Build history of the part. All positions in model axes, mm. A direction names the side the tool comes from. Give positions to 0.01 mm unless a question says otherwise; leave off trailing zeros. Write each loop counter-clockwise with the first axis right and the second up, starting at its lowest first coordinate (ties: lowest second). Pieces come first, ordered by that corner, then holes. Notation, with made-up numbers: (-18, 66) -> (-11, 66) arc R21 cw to (-11, 81) -> close; hole circle Ø7 at (56.5, 64.25). An arc over 180 degrees is marked (long way). Put each result on its own line as item: value. Start each with the question number.
Item 1: Slice it at D-D, the plane x = -12. List the corners of the cut face in (y, z).
Item 2: Tool access for faces 1 (the flat face through (-10.6, 48.1, 2)), 2 (the cylindrical face through (10.28, 45.89, -4.93)), 3 (the cylindrical face through (-29.68, 56.1, -0.87)): list every direction of +Z, -Z, +X, -X, +Y, -Y with a clear straight run to the whole face (end or side of a thin tool).
Item 3: Flat gauge pins, fed straight in: pin 1 Ø7.5 at (x, y) = (-45, 53.5) entering from -Z; pin 2 Ø12 at (y, z) = (23, -4.5) entering from -X; pin 3 Ø4 at (y, z) = (47.5, 6.5) entering from +X; pin 4 Ø2 at (x, y) = (-35.84, 7.78) entering from -Z. Where does each tip first touch, or does it go through?
Item 4: Slice it at B-B, the plane z = -6.5. Give the number of separate pieces and of enclosed holes in the cut face, plus the area to 3 significant figures.
Item 5: Slice it at C-C, the plane y = 42.25. List the corners of the cut face in (x, z).
Item 6: Slice it at A-A, the plane x = -25. List the corners of the cut face in (y, z).
Item 7: Two-plate mould, pull along X, no slides. Class faces 4 (the cylindrical face through (24.295, 39.077, 1.479)), 5 (the flat face through (0, 58, -7)), 6 (the flat face through (48.31, 28.36, 5.07)): pulls with the +X half, pulls with the -X half, needs draft (parallel to the pull), parting line crosses it, or undercut.
Item 8: Drill centre lines: line 1 along X through (y, z) = (8, -7.75); line 2 along Z through (x, y) = (2.5, 16.5); line 3 along Z through (x, y) = (23.5, 20). Where is each one in solid material? Low to high.
```python
from build123d import *

# Parameters (mm, degrees)
BOSS_EXTRUDE2_DEPTH              = 10
FILLET1_R                        = 7.777777778
SKETCH11_R                       = 2.425
SKETCH11_R_2                     = 4
BOSS_EXTRUDE3_DEPTH              = 10
CHAMFER1_SIZE                    = 0.699268119
CHAMFER1_SIZE_2                  = 10
SKETCH11_4_R                     = 3.5
SKETCH11_4_R_2                   = 2.425
BOSS_EXTRUDE4_DEPTH              = 1.5
CBORE_FOR_M3_SHCS2_D             = 3.6
CBORE_FOR_M3_SHCS2_CBORE_D       = 6.5
CBORE_FOR_M3_SHCS2_CBORE_DEPTH   = 8
CUT_EXTRUDE4_DEPTH               = 81.942358333
SKETCH31_W                       = 55
SKETCH31_H                       = 2
BOSS_EXTRUDE5_DEPTH              = 15
FILLET2_R                        = 5
CBORE_FOR_M3_SHCS3_OUTLINE_R     = 1.8
CBORE_FOR_M3_SHCS3_DEPTH         = 10
CBORE_FOR_M3_SHCS3_2_OUTLINE_R   = 3.25
CBORE_FOR_M3_SHCS3_2_OUTLINE_R_2 = 1.8
CBORE_FOR_M3_SHCS3_2_DEPTH       = 3
M3_CLEARANCE_HOLE4_D             = 3.6
SKETCH43_R                       = 4
BOSS_EXTRUDE6_DEPTH              = 10
CBORE_START                      = 2
CBORE_FOR_M3_SHCS4_OUTLINE_R     = 3.25
CBORE_FOR_M3_SHCS4_DEPTH         = 8
CBORE_START_2                    = -10
CBORE_FOR_M3_SHCS4_2_OUTLINE_R   = 1.8
CBORE_FOR_M3_SHCS4_2_DEPTH       = 12


# Read off the part's stored shape, not the designer's step: CBORE for M3 SHCS3, CBORE for M3 SHCS4
with BuildPart() as part:
    # Sketch9 → Boss-Extrude2 (new body)
    with BuildSketch(Plane.XY):
        Polygon((0, 0), (0, 59.5), (-56, 59.5), (-42, 0), align=None)
    boss_extrude2 = extrude(amount=BOSS_EXTRUDE2_DEPTH)

    # Mirror2: Boss-Extrude2 across plane
    add(boss_extrude2.mirror(Plane(origin=(0, 0, 10), x_dir=(0, 0, 1), z_dir=(-1, 0, 0))))

    # Fillet1
    fillet1_edges = [part.edges().sort_by_distance(p)[0] for p in [
        (42, 0, 5),
        (56, 59.5, 5),
        (-42, 0, 5),
        (-56, 59.5, 5),
    ]]
    fillet(fillet1_edges, radius=FILLET1_R)

    # Sketch11 → Boss-Extrude3 (add)
    with BuildSketch(Plane(origin=(0, 0, 0), x_dir=(-1, 0, 0), z_dir=(0, 0, -1))):
        with Locations(Location((-43.410908409, 54.412250943, 0), (0, 0, 180))):
            Circle(SKETCH11_R)
        with Locations(Location((-35.839885988, 7.777777778, 0), (0, 0, 180))):
            Circle(SKETCH11_R_2)
    boss_extrude3 = extrude(amount=BOSS_EXTRUDE3_DEPTH)

    # Chamfer1
    # the kernel refuses this chamfer: 10, 0.699268119 mm, written as the material it takes off along each edge
    with BuildSketch(Plane(origin=(-35.839885988, 0, 10), x_dir=(0, 0.8766829747338895, 0.48106856248536783), z_dir=(1, 0, 0))) as chamfer1_piece_1:
        Polygon((CHAMFER1_SIZE * 0.876682975279, -CHAMFER1_SIZE * 0.481068562785), (-CHAMFER1_SIZE_2 * 0.481068562485, -CHAMFER1_SIZE_2 * 0.876682974734), (0, 0), align=None)
    extrude(amount=71.679771977, mode=Mode.SUBTRACT)
    with BuildSketch(Plane(origin=(35.839885988, 7.777777778, 10), x_dir=(0, -1, 0), z_dir=(-1, 0, 0))) as chamfer1_piece_2:
        Polygon((7.777777778 - CHAMFER1_SIZE, 0), (7.777777778, -CHAMFER1_SIZE_2), (7.777777778, 0), align=None)
    revolve(axis=Axis((35.839885988, 7.777777778, 10), (0, 0, 1)), revolution_arc=76.759480085, mode=Mode.SUBTRACT)
    with BuildSketch(Plane(origin=(-35.839885988, 7.777777778, 10), x_dir=(0, -1, 0), z_dir=(1, 0, 0))) as chamfer1_piece_3:
        Polygon((7.777777778 - CHAMFER1_SIZE, 0), (7.777777778, CHAMFER1_SIZE_2), (7.777777778, 0), align=None)
    revolve(axis=Axis((-35.839885988, 7.777777778, 10), (0, 0, -1)), revolution_arc=76.759480085, mode=Mode.SUBTRACT)
    with BuildSketch(Plane(origin=(53.75077769, 49.940805182, 10), x_dir=(-0.8533782587917171, 0.2007948844215805, 0.4810685624853707), z_dir=(-0.2290393337255473, -0.973417168333576, 0))) as chamfer1_piece_4:
        Polygon((CHAMFER1_SIZE * 0.876682975279, CHAMFER1_SIZE * 0.481068562785), (-CHAMFER1_SIZE_2 * 0.481068562485, CHAMFER1_SIZE_2 * 0.876682974734), (0, 0), align=None)
    extrude(amount=45.144513446, mode=Mode.SUBTRACT)
    with BuildSketch(Plane(origin=(-53.75077769, 49.940805182, 10), x_dir=(0.8533782587917171, 0.2007948844215805, 0.4810685624853707), z_dir=(0.2290393337255473, -0.973417168333576, 0))) as chamfer1_piece_5:
        Polygon((CHAMFER1_SIZE * 0.876682975279, -CHAMFER1_SIZE * 0.481068562785), (-CHAMFER1_SIZE_2 * 0.481068562485, -CHAMFER1_SIZE_2 * 0.876682974734), (0, 0), align=None)
    extrude(amount=45.144513446, mode=Mode.SUBTRACT)
    with BuildSketch(Plane(origin=(46.17975527, 51.722222222, 10), x_dir=(0, 1, 0), z_dir=(-1, 0, 0))) as chamfer1_piece_6:
        Polygon((7.777777778, CHAMFER1_SIZE_2), (7.777777778 - CHAMFER1_SIZE, 0), (7.777777778, 0), align=None)
    revolve(axis=Axis((46.17975527, 51.722222222, 10), (0, 0, -1)), revolution_arc=103.240519915, mode=Mode.SUBTRACT)
    with BuildSketch(Plane(origin=(-46.17975527, 51.722222222, 10), x_dir=(0, 1, 0), z_dir=(1, 0, 0))) as chamfer1_piece_7:
        Polygon((7.777777778, -CHAMFER1_SIZE_2), (7.777777778 - CHAMFER1_SIZE, 0), (7.777777778, 0), align=None)
    revolve(axis=Axis((-46.17975527, 51.722222222, 10), (0, 0, 1)), revolution_arc=103.240519915, mode=Mode.SUBTRACT)
    with BuildSketch(Plane(origin=(-46.17975527, 59.5, 10), x_dir=(0, 0.0026831830283774233, -0.9999964002579389), z_dir=(1, 0, 0))) as chamfer1_piece_8:
        Polygon((CHAMFER1_SIZE_2 * 0.999996400258, -CHAMFER1_SIZE_2 * 0.00268318302838), (-CHAMFER1_SIZE * 0.00268318303005, -CHAMFER1_SIZE * 0.99999640088), (0, 0), align=None)
    extrude(amount=92.359510539, mode=Mode.SUBTRACT)

    # Sketch11<4> → Boss-Extrude4 (add)
    with BuildSketch(Plane(origin=(0, 0, 0), x_dir=(-1, 0, 0), z_dir=(0, 0, -1))):
        with Locations(Location((-43.410908409, 54.412250943, 0), (0, 0, 180))):
            Circle(SKETCH11_4_R)
        with Locations((-43.410908409, 54.412250943)):
            Circle(SKETCH11_4_R_2, mode=Mode.SUBTRACT)
    boss_extrude4 = extrude(amount=BOSS_EXTRUDE4_DEPTH)

    # Mirror3: Boss-Extrude3, Boss-Extrude4 across plane
    add(boss_extrude3.mirror(Plane(origin=(0, 0, 0), x_dir=(0, 0, 1), z_dir=(1, 0, 0))))
    add(boss_extrude4.mirror(Plane(origin=(0, 0, 0), x_dir=(0, 0, 1), z_dir=(1, 0, 0))))

    # CBORE for M3 SHCS2 (through all)
    with Locations(Plane.XY.offset(10)):
        with Locations((35.839885988, 7.777777778)):
            cbore_for_m3_shcs2 = CounterBoreHole(CBORE_FOR_M3_SHCS2_D / 2, CBORE_FOR_M3_SHCS2_CBORE_D / 2, CBORE_FOR_M3_SHCS2_CBORE_DEPTH)

    # Mirror4: CBORE for M3 SHCS2 across plane
    add(cbore_for_m3_shcs2.mirror(Plane(origin=(0, 0, 0), x_dir=(0, 0, 1), z_dir=(1, 0, 0))), mode=Mode.SUBTRACT)

    # Sketch30 → Cut-Extrude4 (cut, through all)
    with BuildSketch(Plane(origin=(0, 0, 0), x_dir=(-1, 0, 0), z_dir=(0, 0, -1))):
        with BuildLine():
            Line((2, 44.5), (2, 19.5))
            ThreePointArc((2, 19.5), (0, 17.5), (-2, 19.5))
            Line((-2, 19.5), (-2, 44.5))
            ThreePointArc((-2, 44.5), (0, 46.5), (2, 44.5))
        make_face()
    extrude(amount=-CUT_EXTRUDE4_DEPTH, mode=Mode.SUBTRACT)

    # Sketch31 → Boss-Extrude5 (add)
    with BuildSketch(Plane(origin=(0, 0, 0), x_dir=(-1, 0, 0), z_dir=(0, 0, -1))):
        with Locations((0, 57)):
            Rectangle(SKETCH31_W, SKETCH31_H)
    extrude(amount=BOSS_EXTRUDE5_DEPTH)

    # Fillet2
    fillet2_edges = [part.edges().sort_by_distance(p)[0] for p in [
        (-27.5, 57, 0),
        (27.5, 57, 0),
        (0, 56, 0),
    ]]
    fillet(fillet2_edges, radius=FILLET2_R)

    # CBORE for M3 SHCS3 outline → CBORE for M3 SHCS3 (cut)
    with BuildSketch(Plane.XY):
        with Locations((25, 17.25)):
            Circle(CBORE_FOR_M3_SHCS3_OUTLINE_R)
        with Locations((-25, 17.25)):
            Circle(CBORE_FOR_M3_SHCS3_OUTLINE_R)
        with Locations((-25, 42.25)):
            Circle(CBORE_FOR_M3_SHCS3_OUTLINE_R)
        with Locations((25, 42.25)):
            Circle(CBORE_FOR_M3_SHCS3_OUTLINE_R)
    extrude(amount=CBORE_FOR_M3_SHCS3_DEPTH, mode=Mode.SUBTRACT)

    # CBORE for M3 SHCS3 2 outline → CBORE for M3 SHCS3 2 (cut)
    # profile 1 of 4: a face of its own
    with BuildSketch(Plane.XY):
        with Locations((25, 17.25)):
            Circle(CBORE_FOR_M3_SHCS3_2_OUTLINE_R)
        with Locations((25, 17.25)):
            Circle(CBORE_FOR_M3_SHCS3_2_OUTLINE_R_2, mode=Mode.SUBTRACT)
    # profile 2 of 4: a face of its own
    with BuildSketch(Plane.XY):
        with Locations((-25, 17.25)):
            Circle(CBORE_FOR_M3_SHCS3_2_OUTLINE_R)
        with Locations((-25, 17.25)):
            Circle(CBORE_FOR_M3_SHCS3_2_OUTLINE_R_2, mode=Mode.SUBTRACT)
    # profile 3 of 4: a face of its own
    with BuildSketch(Plane.XY):
        with Locations((-25, 42.25)):
            Circle(CBORE_FOR_M3_SHCS3_2_OUTLINE_R)
        with Locations((-25, 42.25)):
            Circle(CBORE_FOR_M3_SHCS3_2_OUTLINE_R_2, mode=Mode.SUBTRACT)
    # profile 4 of 4: a face of its own
    with BuildSketch(Plane.XY):
        with Locations((25, 42.25)):
            Circle(CBORE_FOR_M3_SHCS3_2_OUTLINE_R)
        with Locations((25, 42.25)):
            Circle(CBORE_FOR_M3_SHCS3_2_OUTLINE_R_2, mode=Mode.SUBTRACT)
    extrude(amount=CBORE_FOR_M3_SHCS3_2_DEPTH, mode=Mode.SUBTRACT)

    # M3 Clearance Hole4 (through all)
    with Locations(Plane.XY.offset(10)):
        with Locations((-18.75, 52.54589051), (0, 52.54589051), (18.75, 52.54589051)):
            Hole(M3_CLEARANCE_HOLE4_D / 2)

    # Sketch43 → Boss-Extrude6 (add)
    with BuildSketch(Plane(origin=(0, 0, 0), x_dir=(-1, 0, 0), z_dir=(0, 0, -1))):
        with BuildLine():
            ThreePointArc((8.291900756, 51), (11.23593095, 45.57365329), (16, 49.5))
            ThreePointArc((16, 49.5), (15.92634671, 50.26406905), (15.708099244, 51))
            Line((15.708099244, 51), (8.291900756, 51))
        make_face()
        with BuildLine():
            Line((8.291900756, 51), (15.708099244, 51))
            ThreePointArc((15.708099244, 51), (12, 53.5), (8.291900756, 51))
        make_face()
        with Locations(Location((-12, 49.5, 0), (0, 0, 157.975687163))):
            Circle(SKETCH43_R)
    extrude(amount=BOSS_EXTRUDE6_DEPTH)

    # CBORE for M3 SHCS4 outline → CBORE for M3 SHCS4 (cut)
    with BuildSketch(Plane.XY.offset(CBORE_START)):
        with Locations((-12, 49.5)):
            Circle(CBORE_FOR_M3_SHCS4_OUTLINE_R)
        with Locations((12, 49.5)):
            Circle(CBORE_FOR_M3_SHCS4_OUTLINE_R)
    extrude(amount=CBORE_FOR_M3_SHCS4_DEPTH, mode=Mode.SUBTRACT)

    # CBORE for M3 SHCS4 2 outline → CBORE for M3 SHCS4 2 (cut)
    with BuildSketch(Plane.XY.offset(CBORE_START_2)):
        with Locations((-12, 49.5)):
            Circle(CBORE_FOR_M3_SHCS4_2_OUTLINE_R)
        with Locations((12, 49.5)):
            Circle(CBORE_FOR_M3_SHCS4_2_OUTLINE_R)
    extrude(amount=CBORE_FOR_M3_SHCS4_2_DEPTH, mode=Mode.SUBTRACT)


solid = part.part
```
Values follow:
1. outline: (0, 0) -> (45.5, 0) -> (45.5, -10) -> (47.7, -10) -> (47.7, 2) -> (46.25, 2) -> (46.25, 10) -> (0.7, 10) -> close; (51.3, -10) -> (53.5, -10) -> (53.5, -0.67) arc R5 cw to (56, -5) -> (56, -15) -> (58, -15) -> (58, 0) -> (59.5, 0) -> (58.8, 10) -> (52.75, 10) -> (52.75, 2) -> (51.3, 2) -> close
2. face 1: +Z
2. face 2: -Z
2. face 3: -Z, +Y
3. pin 1: z = -10
3. pin 2: x = -48.35
3. pin 3: x = 53.2
3. pin 4: through
4. separate pieces: 7
4. enclosed holes: 4
4. area: 307 mm2
5. outline: (-51.94, 0) -> (-28.25, 0) -> (-28.25, 3) -> (-26.8, 3) -> (-26.8, 10) -> (-51.22, 10) -> close; (-23.2, 3) -> (-21.75, 3) -> (-21.75, 0) -> (-2, 0) -> (-2, 10) -> (-23.2, 10) -> close; (2, 0) -> (21.75, 0) -> (21.75, 3) -> (23.2, 3) -> (23.2, 10) -> (2, 10) -> close; (26.8, 3) -> (28.25, 3) -> (28.25, 0) -> (51.94, 0) -> (51.22, 10) -> (26.8, 10) -> close
6. outline: (0, 0) -> (14, 0) -> (14, 3) -> (15.45, 3) -> (15.45, 10) -> (0.7, 10) -> close; (19.05, 3) -> (20.5, 3) -> (20.5, 0) -> (39, 0) -> (39, 3) -> (40.45, 3) -> (40.45, 10) -> (19.05, 10) -> close; (44.05, 3) -> (45.5, 3) -> (45.5, 0) -> (51, 0) arc R5 cw to (56, -5) -> (56, -15) -> (58, -15) -> (58, 0) -> (59.5, 0) -> (58.8, 10) -> (44.05, 10) -> close
7. face 4: undercut
7. face 5: needs draft
7. face 6: pulls with the +X half
8. line 1: -39.83 to -37.63, -34.05 to -31.85, 31.85 to 34.05, 37.63 to 39.83
8. line 2: 0 to 10
8. line 3: 3 to 10
